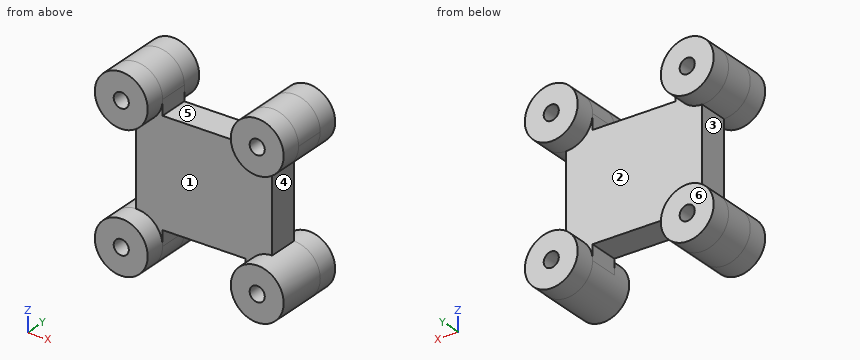
```python
from build123d import *

# Parameters (mm, degrees)
SKETCH1_W           = 22
SKETCH1_H           = 28
BOSS_EXTRUDE1_DEPTH = 8
SKETCH2_R           = 2
CUT_EXTRUDE1_DEPTH  = 37.249137921
SKETCH5_R           = 7
SKETCH5_R_2         = 2
BOSS_EXTRUDE3_DEPTH = 5.5


with BuildPart() as part:
    # Sketch1 → Boss-Extrude1 (new body)
    with BuildSketch(Plane(origin=(0, 0, 0), x_dir=(1, 0, 0), z_dir=(0, 1, 0))):
        with BuildLine():
            ThreePointArc((-18, 11), (-13.050252532, 13.050252532), (-11, 18))
            Line((-11, 18), (-18, 18))
            Line((-18, 18), (-18, 11))
        make_face()
        with BuildLine():
            Line((-18, 18), (-11, 18))
            ThreePointArc((-11, 18), (-22.949747468, 22.949747468), (-18, 11))
            Line((-18, 11), (-18, 18))
        make_face()
        with BuildLine():
            Line((-11, -18), (-11, -14))
            Line((-11, -14), (-11, 14))
            Line((-11, 14), (-11, 18))
            ThreePointArc((-11, 18), (-13.050252532, 13.050252532), (-18, 11))
            Line((-18, 11), (-18, -11))
            ThreePointArc((-18, -11), (-13.050252532, -13.050252532), (-11, -18))
        make_face()
        with BuildLine():
            ThreePointArc((-18, -11), (-22.949747468, -22.949747468), (-11, -18))
            Line((-11, -18), (-18, -18))
            Line((-18, -18), (-18, -11))
        make_face()
        with BuildLine():
            Line((-18, -18), (-11, -18))
            ThreePointArc((-11, -18), (-13.050252532, -13.050252532), (-18, -11))
            Line((-18, -11), (-18, -18))
        make_face()
        Rectangle(SKETCH1_W, SKETCH1_H)
        with BuildLine():
            ThreePointArc((18, -11), (13.050252532, -13.050252532), (11, -18))
            Line((11, -18), (18, -18))
            Line((18, -18), (18, -11))
        make_face()
        with BuildLine():
            Line((18, -18), (11, -18))
            ThreePointArc((11, -18), (18, -25), (25, -18))
            ThreePointArc((25, -18), (22.949747468, -13.050252532), (18, -11))
            Line((18, -11), (18, -18))
        make_face()
        with BuildLine():
            Line((11, 14), (11, -14))
            Line((11, -14), (11, -18))
            ThreePointArc((11, -18), (13.050252532, -13.050252532), (18, -11))
            Line((18, -11), (18, 11))
            ThreePointArc((18, 11), (13.050252532, 13.050252532), (11, 18))
            Line((11, 18), (11, 14))
        make_face()
        with BuildLine():
            ThreePointArc((25, 18), (18, 25), (11, 18))
            Line((11, 18), (18, 18))
            Line((18, 18), (18, 11))
            ThreePointArc((18, 11), (22.949747468, 13.050252532), (25, 18))
        make_face()
        with BuildLine():
            Line((18, 18), (11, 18))
            ThreePointArc((11, 18), (13.050252532, 13.050252532), (18, 11))
            Line((18, 11), (18, 18))
        make_face()
    extrude(amount=BOSS_EXTRUDE1_DEPTH)

    # Sketch2 → Cut-Extrude1 (cut, through all)
    with BuildSketch(Plane(origin=(0, 8, 0), x_dir=(1, 0, 0), z_dir=(0, 1, 0))):
        with Locations(Location((-18, 18, 0), (0, 0, 270))):
            Circle(SKETCH2_R)
        with Locations(Location((-18, -18, 0), (0, 0, 270))):
            Circle(SKETCH2_R)
        with Locations(Location((18, -18, 0), (0, 0, 270))):
            Circle(SKETCH2_R)
        with Locations(Location((18, 18, 0), (0, 0, 270))):
            Circle(SKETCH2_R)
    extrude(amount=-CUT_EXTRUDE1_DEPTH, mode=Mode.SUBTRACT)

    # Sketch5 → Boss-Extrude3 (add)
    # profile 1 of 4: a face of its own
    with BuildSketch(Plane.XZ):
        with Locations(Location((-18, 18, 0), (0, 0, 270))):
            Circle(SKETCH5_R)
        with Locations(Location((-18, 18, 0), (0, 0, 90))):
            Circle(SKETCH5_R_2, mode=Mode.SUBTRACT)
    # profile 2 of 4: a face of its own
    with BuildSketch(Plane.XZ):
        with Locations(Location((18, 18, 0), (0, 0, 270))):
            Circle(SKETCH5_R)
        with Locations(Location((18, 18, 0), (0, 0, 90))):
            Circle(SKETCH5_R_2, mode=Mode.SUBTRACT)
    # profile 3 of 4: a face of its own
    with BuildSketch(Plane.XZ):
        with Locations(Location((18, -18, 0), (0, 0, 270))):
            Circle(SKETCH5_R)
        with Locations(Location((18, -18, 0), (0, 0, 90))):
            Circle(SKETCH5_R_2, mode=Mode.SUBTRACT)
    # profile 4 of 4: a face of its own
    with BuildSketch(Plane.XZ):
        with Locations(Location((-18, -18, 0), (0, 0, 270))):
            Circle(SKETCH5_R)
        with Locations(Location((-18, -18, 0), (0, 0, 90))):
            Circle(SKETCH5_R_2, mode=Mode.SUBTRACT)
    boss_extrude3 = extrude(amount=BOSS_EXTRUDE3_DEPTH)

    # Mirror1: Boss-Extrude3 across plane
    add(boss_extrude3.mirror(Plane.ZX.offset(4)))


solid = part.part
```
Geometry: final body of the model. Coordinates: model frame, mm. Face numbers are marked on the shaded views. A direction names the side the tool comes from. Round coordinates to 2 decimals unless told otherwise and drop trailing zeros. Write each loop counter-clockwise with the first axis right and the second up, starting at its lowest first coordinate (ties: lowest second). Pieces come first, ordered by that corner, then holes.
Item 1: Mould query, pull axis X, two halves, no side actions, for the marked faces 4, 5 and 6. Classes: +X half, -X half, draft (parallel to the pull), parting line (faces both ways), or undercut.
Item 2: Pin query (flat end, axial travel): P1, Ø5, axis at y = 9.5, z = -4.5, coming from the -X side; P2, Ø4, axis at y = 9, z = 12, coming from the -X side; P3, Ø1, axis at x = 6, z = -4.5, coming from the +Y side; P4, Ø3.5, axis at x = 18, z = 18, coming from the -Y side. Return the tip coordinate at first contact, or that it passes through.
Item 3: Section query D-D (z = -15). Return loops of the section in (x, y).
Item 4: Section query C-C (x = -21). Return loops of the section in (y, z).
Item 5: Set-up query: the marked faces 1, 2 and 3. Return all of +Z, -Z, +X, -X, +Y, -Y with unobstructed straight access to the full face (end or side cutting, diameter ignored); none if empty.
Item 6: Section query B-B (y = 6.25). Return loops of the section in (x, z), plus the area to 3 significant figures.
Item 7: Section query A-A (y = 9.5). Return loops of the section in (x, z).
Item 8: Material intervals for L1, parallel to X at y = -3.6, z = -18; L2, parallel to Z at x = -1, y = 1.5, sorted ascending.
Completed:
1. face 4: +X half
1. face 5: undercut
1. face 6: draft
2. P1: stops at x = -18
2. P2: stops at x = -23.74
2. P3: stops at y = 8
2. P4: passes through
3. outline: (-24.32, -5.5) - (-11.68, -5.5) - (-11.68, 0) - (-11, 0) - (-11, 8) - (-11.68, 8) - (-11.68, 13.5) - (-24.32, 13.5) - close; (11, 0) - (11.68, 0) - (11.68, -5.5) - (24.32, -5.5) - (24.32, 13.5) - (11.68, 13.5) - (11.68, 8) - (11, 8) - close
4. outline: (-5.5, -24.32) - (13.5, -24.32) - (13.5, -11.68) - (-5.5, -11.68) - close; (-5.5, 11.68) - (13.5, 11.68) - (13.5, 24.32) - (-5.5, 24.32) - close
5. face 1: -Y
5. face 2: +Y
5. face 3: -X, +Y, -Y
6. outline: (-18, -11) arc R7 ccw (long way) to (-11, -18) - (-11, -14) - (11, -14) - (11, -18) arc R7 ccw (long way) to (18, -11) - (18, 11) arc R7 ccw (long way) to (11, 18) - (11, 14) - (-11, 14) - (-11, 18) arc R7 ccw (long way) to (-18, 11) - close; hole circle Ø4 at (-18, -18); hole circle Ø4 at (-18, 18); hole circle Ø4 at (18, -18); hole circle Ø4 at (18, 18)
6. area: 1,530 mm2
7. outline: circle Ø14 at (-18, -18); circle Ø14 at (-18, 18); circle Ø14 at (18, -18); circle Ø14 at (18, 18); hole circle Ø4 at (-18, -18); hole circle Ø4 at (-18, 18); hole circle Ø4 at (18, -18); hole circle Ø4 at (18, 18)
8. L1: x = -25 to -20, -16 to -11, 11 to 16, 20 to 25
8. L2: z = -14 to 14
